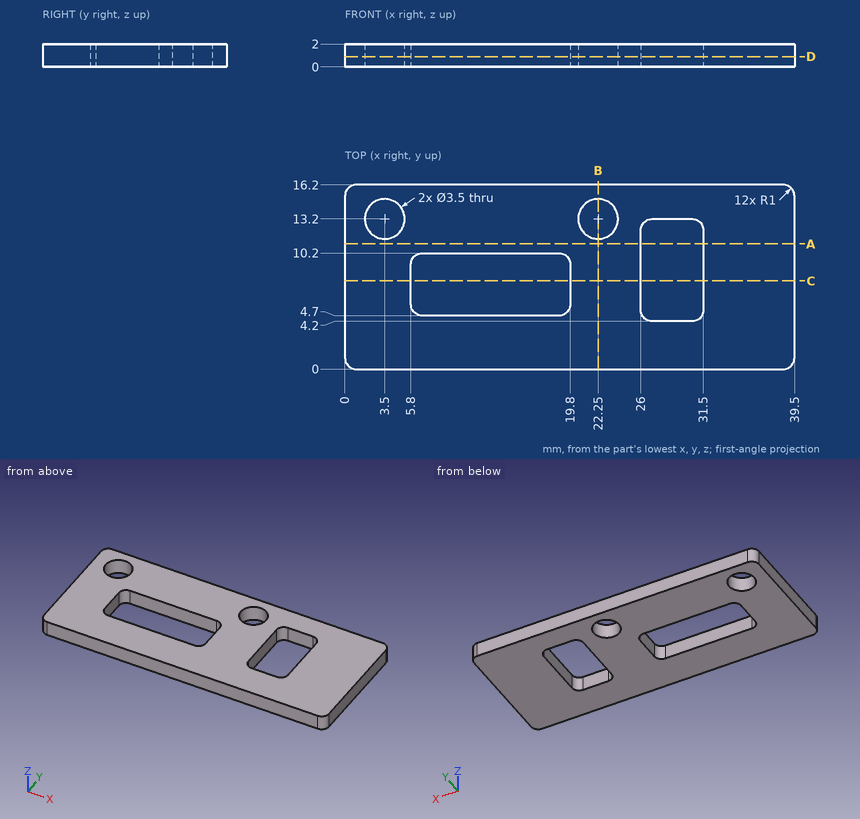
Here's the drawing with two shaded views (mm, measured from the low corner). I have some questions. Round coordinates to 2 decimals unless told otherwise and drop trailing zeros. Loops run counter-clockwise (first coordinate to the right, second up) from the corner with the lowest first, then second, coordinate; pieces in that order, holes last. Notation, with made-up numbers: (-36.75, -15.5) -> (-9.75, -15.5) arc R22 cw to (-9.75, 14.5) -> close; hole circle Ø7 at (26.5, 52). An arc over 180 degrees is marked (long way). Answer as CSV lines item,"result". Start each with the question number.
1. I need wall thicknesses on probe 1 along X at (y, z) = (8.5, 1.7); probe 2 along Y at (x, z) = (18, 0.45); probe 3 along Y at (x, z) = (22.25, 0.9). Which ranges of each line are inside material? Lowest first, please. Write a range as from..to.
2. Imagine slicing it at D-D on z = 0.9. Write out the boundary of the cut face in (x, y).
3. Imagine slicing it at C-C on y = 7.75. Write out the boundary of the cut face in (x, z).
4. Imagine slicing it at A-A on y = 11. Write out the boundary of the cut face in (x, z).
5. Imagine slicing it at B-B on x = 22.25. Write out the boundary of the cut face in (y, z), plus the area to 3 significant figures.
Solution:
1,probe 1,"0..5.8, 19.8..26, 31.5..39.5"
1,probe 2,"0..4.7, 10.2..16.2"
1,probe 3,"0..11.45, 14.95..16.2"
2,outline,"(0, 1) arc R1 ccw to (1, 0) -> (38.5, 0) arc R1 ccw to (39.5, 1) -> (39.5, 15.2) arc R1 ccw to (38.5, 16.2) -> (1, 16.2) arc R1 ccw to (0, 15.2) -> close; hole circle Ø3.5 at (3.5, 13.2); hole (5.8, 5.7) arc R1 ccw to (6.8, 4.7) -> (18.8, 4.7) arc R1 ccw to (19.8, 5.7) -> (19.8, 9.2) arc R1 ccw to (18.8, 10.2) -> (6.8, 10.2) arc R1 ccw to (5.8, 9.2) -> close; hole circle Ø3.5 at (22.25, 13.2); hole (26, 5.2) arc R1 ccw to (27, 4.2) -> (30.5, 4.2) arc R1 ccw to (31.5, 5.2) -> (31.5, 12.2) arc R1 ccw to (30.5, 13.2) -> (27, 13.2) arc R1 ccw to (26, 12.2) -> close"
3,outline,"(0, 0) -> (5.8, 0) -> (5.8, 2) -> (0, 2) -> close; (19.8, 0) -> (26, 0) -> (26, 2) -> (19.8, 2) -> close; (31.5, 0) -> (39.5, 0) -> (39.5, 2) -> (31.5, 2) -> close"
4,outline,"(0, 0) -> (26, 0) -> (26, 2) -> (0, 2) -> close; (31.5, 0) -> (39.5, 0) -> (39.5, 2) -> (31.5, 2) -> close"
5,outline,"(0, 0) -> (11.45, 0) -> (11.45, 2) -> (0, 2) -> close; (14.95, 0) -> (16.2, 0) -> (16.2, 2) -> (14.95, 2) -> close"
5,area,"25.4 mm²"
